Verification items for the finished model (mm, model axes). Coordinates: 2 decimals unless noted, no trailing zeros. Loops run counter-clockwise (first coordinate to the right, second up) from the corner with the lowest first, then second, coordinate; pieces in that order, holes last. Notation, with made-up numbers: (62.25, 15) -> (116.25, 15) arc R9 cw to (116.25, 21) -> close; hole circle Ø10 at (41.5, 15). An arc over 180 degrees is marked (long way). Write item = value, one per line.
```python
from build123d import *

# Parameters (mm, degrees)
F0_W     = 22
F0_H     = 22
F1_DEPTH = 22
F5_DEPTH = 22.001


with BuildPart() as f1:
    # F0 (on Front) → F1 (new body)
    with BuildSketch(Plane.XZ):
        with Locations((12.5, 12.5)):
            Rectangle(F0_W, F0_H)
    extrude(amount=F1_DEPTH)

    # F2 (on face) → F5 (cut, through all)
    with BuildSketch(Plane.XZ.offset(22)):
        with BuildLine():
            Line((15.3284271247, 15.3284271247), (12.5, 12.5))
            Line((12.5, 12.5), (15.3284271247, 9.6715728753))
            ThreePointArc((15.3284271247, 9.6715728753), (16.19551813, 10.9692662705), (16.5, 12.5))
            ThreePointArc((16.5, 12.5), (16.19551813, 14.0307337295), (15.3284271247, 15.3284271247))
        make_face()
        with BuildLine():
            ThreePointArc((15.3284271247, 15.3284271247), (12.5, 16.5), (9.6715728753, 15.3284271247))
            Line((9.6715728753, 15.3284271247), (12.5, 12.5))
            Line((12.5, 12.5), (15.3284271247, 15.3284271247))
        make_face()
        with BuildLine():
            Line((12.5, 12.5), (9.6715728753, 15.3284271247))
            ThreePointArc((9.6715728753, 15.3284271247), (8.5, 12.5), (9.6715728753, 9.6715728753))
            Line((9.6715728753, 9.6715728753), (12.5, 12.5))
        make_face()
        with BuildLine():
            Line((15.3284271247, 9.6715728753), (12.5, 12.5))
            Line((12.5, 12.5), (9.6715728753, 9.6715728753))
            ThreePointArc((9.6715728753, 9.6715728753), (12.5, 8.5), (15.3284271247, 9.6715728753))
        make_face()
    extrude(amount=-F5_DEPTH, mode=Mode.SUBTRACT)


solid = f1.part
```
1) Sectioned sample at C-C, the plane z = 13.75. Record the cut outline in (x, y).
Ans:
outline = (1.5, -22) -> (8.7, -22) -> (8.7, 0) -> (1.5, 0) -> close; (16.3, -22) -> (23.5, -22) -> (23.5, 0) -> (16.3, 0) -> close
2) Depth check by flat-ended pin: pin 1 Ø12 at (x, z) = (12, 17) entering from +Y. Enter the tip coordinate at first touch or a pass-through.
Ans:
pin_1 = 0
3) Material ranges on line 1 (X direction, y = -4.75, z = 15); line 2 (X direction, y = -4.5, z = 14); line 3 (Z direction, x = 14.5, y = -12.5), recorded low to high.
Ans:
line_1 = 1.5 to 9.38, 15.62 to 23.5
line_2 = 1.5 to 8.79, 16.21 to 23.5
line_3 = 1.5 to 9.04, 15.96 to 23.5
4) Sectioned sample at B-B, the plane x = 14.25. Record the cut outline in (y, z).
Ans:
outline = (-22, 1.5) -> (0, 1.5) -> (0, 8.9) -> (-22, 8.9) -> close; (-22, 16.1) -> (0, 16.1) -> (0, 23.5) -> (-22, 23.5) -> close
5) Sectioned sample at A-A, the plane y = -8.5. Record the cut outline in (x, z).
Ans:
outline = (1.5, 1.5) -> (23.5, 1.5) -> (23.5, 23.5) -> (1.5, 23.5) -> close; hole circle Ø8 at (12.5, 12.5)
